```python
from build123d import *

# Parameters (mm, degrees)
F2_R = 4.486307
F3_R = 0.215658
F4_R = 2.5393


with BuildPart() as f1:
    # F0 (on Front) → F1 (revolve)
    with BuildSketch(Plane.XZ):
        Polygon((-8.137501, 0), (0, 0), (0, 17.0625), (-1.137501, 17.0625), (-3.762501, 15.8375), (-5.6875, 11.2875), (-5.3375, 9.5375), (-6.562501, 9.1875), align=None)
    revolve(axis=Axis((0, 0, 8.53125), (0, 0, -1)))

    # F2
    f2_edges = [f1.edges().sort_by_distance(p)[0] for p in [
        (1.137501, 0, 17.0625),
        (3.762501, 0, 15.8375),
        (-2.450001, 0, 16.45),
    ]]
    fillet(f2_edges, radius=F2_R)

    # F3
    f3_edges = [f1.edges().sort_by_distance(p)[0] for p in [
        (-5.060953, 0, 12.768431),
        (4.434386, 0, 14.249362),
        (5.6875, 0, 11.2875),
    ]]
    fillet(f3_edges, radius=F3_R)

    # F4
    f4_edges = [f1.edges().sort_by_distance(p)[0] for p in [
        (8.137501, 0, 0),
    ]]
    fillet(f4_edges, radius=F4_R)


solid = f1.part
```
For this review, take the finished solid that the model builds, in its own axes (mm). Round coordinates to 2 decimals unless told otherwise and drop trailing zeros. Write each loop counter-clockwise with the first axis right and the second up, starting at its lowest first coordinate (ties: lowest second). Pieces come first, ordered by that corner, then holes. Notation, with made-up numbers: (28, 13.5) - (76, 13.5) arc R13 cw to (76, 26.5) - close; hole circle Ø4 at (25, 18). An arc over 180 degrees is marked (long way). Write each question's results on one line, items separated by ' | '.
Item 1: Take a section at A-A on z = 1.5. State the section outline as (x, y) points.
Calculated:
outline: circle Ø14.89 at (0, 0)
Item 2: Take a section at B-B on z = 13. State the section outline as (x, y) points, then the cut area to 3 significant figures.
Calculated:
outline: circle Ø9.93 at (0, 0) | area: 77.4 mm^2
Item 3: For pin 1 (8 mm diameter, centred on x = 3.5, z = 12, fed in from -Y); pin 2 (4 mm diameter, centred on x = -2, z = 5.5, fed in from -Y); pin 3 (2 mm diameter, centred on x = -5, z = 11, fed in from -Y), all flat-tipped, find the tip position at first contact; note any pin that passes through.
Calculated:
pin 1: stops at y = -6.54 | pin 2: stops at y = -7.43 | pin 3: stops at y = -4
Item 4: To check wall thickness, follow line 1 along X through (y, z) = (-3.75, 14.25); line 2 along Y through (x, z) = (-3, 10.5); line 3 along Y through (x, z) = (5.5, 1.75). State the ranges of each line that lie inside material, in increasing order. Write a range as from..to.
Calculated:
line 1: x = -2.37..2.37 | line 2: y = -4.65..4.65 | line 3: y = -5.16..5.16
